Geometry: final body of the model. Coordinates: model frame, mm. Round coordinates to 2 decimals unless told otherwise and drop trailing zeros. Write each loop counter-clockwise with the first axis right and the second up, starting at its lowest first coordinate (ties: lowest second). Pieces come first, ordered by that corner, then holes. Notation, with made-up numbers: (13.5, 84.5) - (65.5, 84.5) arc R16 ccw to (65.5, 104.5) - close; hole circle Ø10 at (-27, -9). An arc over 180 degrees is marked (long way). Use a Markdown table: item, result. Add a question column.
```python
from build123d import *

# Parameters (mm, degrees)
F0_W     = 30
F0_H     = 30
F1_DEPTH = 10
F2_R     = 4.99999


# Not quite as in the source:
# - a fillet or chamfer is up to 0.001 mm smaller than in the source, because OpenCascade refuses the exact size


with BuildPart() as f1:
    # F0 (on Top) → F1 (new body)
    with BuildSketch(Plane.XY):
        Polygon((0, 28.652399919), (-35, 58.652399919), (-35, 28.652399919), align=None)
        with Locations((-50, 43.652399919)):
            Rectangle(F0_W, F0_H)
    extrude(amount=F1_DEPTH)

    # F2 (radius 5 in the source; OpenCascade refuses exactly that, so slightly less here)
    f2_edges = [f1.edges().sort_by_distance(p)[0] for p in [
        (-17.5, 43.6524, 10),
        (-50, 58.6524, 10),
        (-65, 43.6524, 10),
        (-32.5, 28.6524, 10),
        (-32.5, 28.6524, 0),
        (-65, 43.6524, 0),
        (-50, 58.6524, 0),
        (-17.5, 43.6524, 0),
        (-35, 58.6524, 5),
        (0, 28.6524, 5),
    ]]
    fillet(f2_edges, radius=F2_R)


solid = f1.part
```
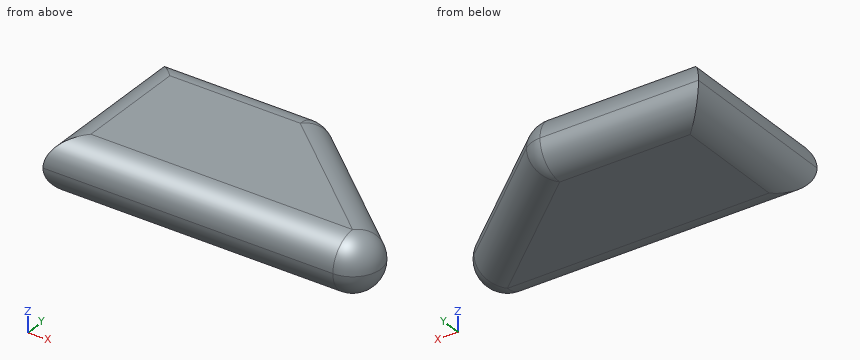
1) Section B-B, the plane z = 5.75. Return the cut outline in (x, y), then the cut area to 3 significant figures.
2) Material intervals for L1, parallel to Y at x = -19.5, z = 4.5; L2, parallel to X at y = 53.5, z = 3; L3, parallel to X at y = 36.5, z = 6.75, sorted ascending. Write a range as from..to.
3) Pin query (flat end, axial travel): P1, Ø1.5, axis at x = -29.5, z = 3, coming from the -Y side; P2, Ø6, axis at x = -27, z = 5, coming from the +Y side; P3, Ø2, axis at y = 37, z = 5.5, coming from the +X side. Return the tip coordinate at first contact, or that it passes through.
4) Section C-C, the plane z = 1. Return the cut outline in (x, y).
Output values:
| question | item | result |
|---|---|---|
| 1 | outline | (-64.94, 28.71) - (-13.52, 28.71) arc R4.94 ccw to (-10.3, 37.41) - (-33.63, 57.41) arc R4.94 ccw to (-36.85, 58.6) - (-64.94, 58.6) - close |
| 1 | area | 1,380 mm^2 |
| 2 | L1 | y = 28.68..45.33 |
| 2 | L2 | x = -64.58..-29.63 |
| 2 | L3 | x = -64.68..-9.8 |
| 3 | P1 | stops at y = 28.81 |
| 3 | P2 | stops at y = 54.37 |
| 3 | P3 | stops at x = -9.12 |
| 4 | outline | (-63, 30.65) - (-13.52, 30.65) arc R3 ccw to (-11.56, 35.93) - (-34.9, 55.93) arc R3 ccw to (-36.85, 56.65) - (-63, 56.65) - close |
